Input: part model. Units: mm. Frame: model coordinates. Face numbers are marked on the shaded views. Coordinates: 2 decimals unless noted, no trailing zeros. Write each loop counter-clockwise with the first axis right and the second up, starting at its lowest first coordinate (ties: lowest second). Pieces come first, ordered by that corner, then holes. Notation, with made-up numbers: (30, 56.5) - (75, 56.5) arc R26 cw to (75, 70.5) - close; hole circle Ø5 at (-7, -22). An arc over 180 degrees is marked (long way). Use CSV: the item, a comma, the result in double quotes.
```python
from build123d import *

# Parameters (mm, degrees)
SKETCH1_R                = 4
SKETCH1_W                = 28.8
SKETCH1_H                = 60
BOSS_EXTRUDE1_DEPTH      = 6.35
F_5_16_CLEARANCE_HOLE1_D = 8.2042
FILLET1_R                = 10


with BuildPart() as part:
    # Sketch1 → Boss-Extrude1 (new body)
    with BuildSketch(Plane(origin=(0, 0, 0), x_dir=(0, 0, -1), z_dir=(1, 0, 0))):
        with Locations((0, -6)):
            Circle(SKETCH1_R)
        with Locations((0, 8.53)):
            Circle(SKETCH1_R)
        Rectangle(SKETCH1_W, SKETCH1_H)
        with Locations((0, -6)):
            Circle(SKETCH1_R, mode=Mode.SUBTRACT)
        with Locations((0, 8.53)):
            Circle(SKETCH1_R, mode=Mode.SUBTRACT)
    extrude(amount=BOSS_EXTRUDE1_DEPTH)

    # 5/16 Clearance Hole1 (through all)
    with Locations(Plane.ZY):
        with Locations((0, 8.53), (0, -6)):
            Hole(F_5_16_CLEARANCE_HOLE1_D / 2)

    # Fillet1
    fillet1_edges = [part.edges().sort_by_distance(p)[0] for p in [
        (3.175, 30, 14.4),
        (3.175, 30, -14.4),
        (3.175, -30, -14.4),
        (3.175, -30, 14.4),
    ]]
    fillet(fillet1_edges, radius=FILLET1_R)


solid = part.part
```
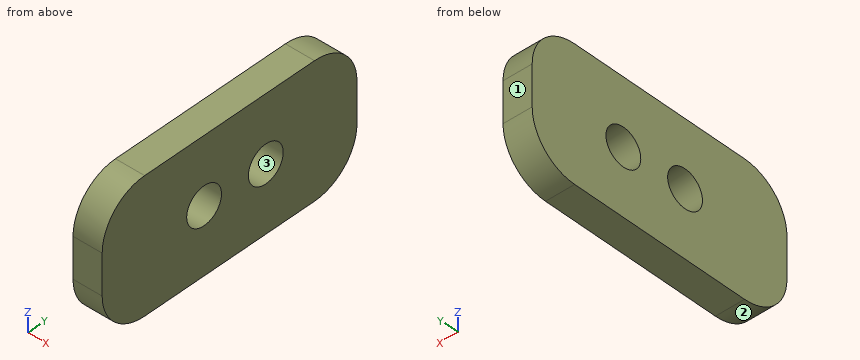
(1) Ray query, probe 1 along Y at (x, z) = (2.5, 0); probe 2 along Y at (x, z) = (5.5, -2.5); probe 3 along Z at (x, y) = (4.5, 8). Return the intervals inside material, ascending. Write a range as from..to.
Check values:
probe 1,"-30..-10.1, -1.9..4.43, 12.63..30"
probe 2,"-30..-9.25, -2.75..5.28, 11.78..30"
probe 3,"-14.4..-4.07, 4.07..14.4"
(2) Cut plane B-B on z = 0. Return loops of the section in (x, y).
Check values:
outline,"(0, -30) - (6.35, -30) - (6.35, -10.1) - (0, -10.1) - close; (0, -1.9) - (6.35, -1.9) - (6.35, 4.43) - (0, 4.43) - close; (0, 12.63) - (6.35, 12.63) - (6.35, 30) - (0, 30) - close"
(3) Cut plane D-D on z = -3.25. Return loops of the section in (x, y), and give its area (3 significant figures).
Check values:
outline,"(0, -30) - (6.35, -30) - (6.35, -8.5) - (0, -8.5) - close; (0, -3.5) - (6.35, -3.5) - (6.35, 6.03) - (0, 6.03) - close; (0, 11.03) - (6.35, 11.03) - (6.35, 30) - (0, 30) - close"
area,"317 mm^2"
(4) Cut plane A-A on y = 8.53. Return loops of the section in (x, z), and give its area (3 significant figures).
Check values:
outline,"(0, -14.4) - (6.35, -14.4) - (6.35, -4.1) - (0, -4.1) - close; (0, 4.1) - (6.35, 4.1) - (6.35, 14.4) - (0, 14.4) - close"
area,"131 mm^2"
(5) Cut plane C-C on x = 2. Return loops of the section in (y, z), and give its area (3 significant figures).
Check values:
outline,"(-30, -4.4) arc R10 ccw to (-20, -14.4) - (20, -14.4) arc R10 ccw to (30, -4.4) - (30, 4.4) arc R10 ccw to (20, 14.4) - (-20, 14.4) arc R10 ccw to (-30, 4.4) - close; hole circle Ø8.2 at (-6, 0); hole circle Ø8.2 at (8.53, 0)"
area,"1,540 mm^2"
(6) Draft query along Y for the marked faces 1, 2 and 3. Return one class per face: pulls with the +Y half, pulls with the -Y half, needs draft (parallel to the pull), parting line crosses it, or undercut.
Check values:
face 1,"pulls with the +Y half"
face 2,"pulls with the -Y half"
face 3,"undercut"
(7) Pin query (flat end, axial travel): pin 1 Ø2 at (x, z) = (3.5, -7) entering from -Y. Return the tip coordinate at first contact, or that it passes through.
Check values:
pin 1,"y = -29.87"
